The drawing under review shows one solid part. Ordinate dimensions are in mm from its lowest x, y, z. A direction names the side the tool comes from. Give positions to 0.01 mm unless a question says otherwise; leave off trailing zeros. Loops run counter-clockwise (first coordinate to the right, second up) from the corner with the lowest first, then second, coordinate; pieces in that order, holes last. Notation, with made-up numbers: (14, 46.5) -> (49, 46.5) arc R28 cw to (49, 76.5) -> close; hole circle Ø11 at (56, 83). An arc over 180 degrees is marked (long way). Answer in a Markdown table with one row per item. Add a question column.
(1) Draft analysis for pull direction X (two halves, no side actions). For the marked faces 3, 4 and 5, state which applies: +X half, -X half, draft (parallel to the pull), parting line (faces both ways), or undercut.
(2) Consider section B-B on x = 14.5. Write out the cut boundary in (y, z), then the cut area to 3 significant figures.
(3) Consider section A-A on z = 25. Write out the cut boundary in (x, y), then the cut area to 3 significant figures.
(4) For line 1 (Z direction, x = 9.5, y = 0.4); line 2 (Y direction, x = 7.5, z = 17); line 3 (X direction, y = 0.25, z = 25), list the stretches that pass through material, from the lowest coordinate up.
(5) For the marked faces 1 and 2, list the 3-axis set-ups (+Z, -Z, +X, -X, +Y, -Y) from which the entire face can be reached by the end or side of a thin tool; tool diameter is ignored.
(6) Consider section D-D on x = 9.5. Write out the cut boundary in (y, z).
(7) For pin 1 (8.5 mm diameter, centred on y = 6, z = 12.5, fed in from -X); pin 2 (5 mm diameter, centred on x = 5, y = 9, fed in from -Z), all flat-tipped, find the tip position at first contact; note any pin that passes through.
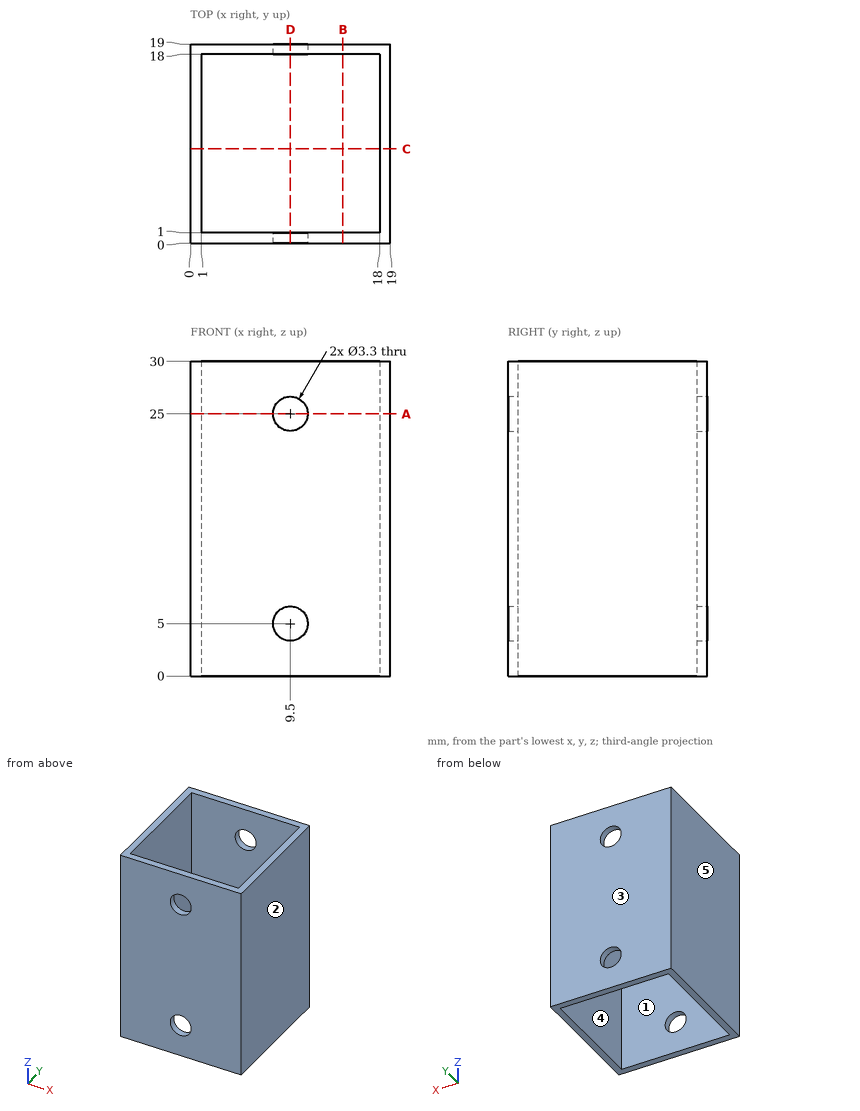
Values follow:
| question | item | result |
|---|---|---|
| 1 | face 3 | draft |
| 1 | face 4 | undercut |
| 1 | face 5 | -X half |
| 2 | outline | (0, 0) -> (1, 0) -> (1, 30) -> (0, 30) -> close; (18, 0) -> (19, 0) -> (19, 30) -> (18, 30) -> close |
| 2 | area | 60.0 mm2 |
| 3 | outline | (0, 0) -> (7.85, 0) -> (7.85, 1) -> (1, 1) -> (1, 18) -> (7.85, 18) -> (7.85, 19) -> (0, 19) -> close; (11.15, 0) -> (19, 0) -> (19, 19) -> (11.15, 19) -> (11.15, 18) -> (18, 18) -> (18, 1) -> (11.15, 1) -> close |
| 3 | area | 65.4 mm2 |
| 4 | line 1 | 0 to 3.35, 6.65 to 23.35, 26.65 to 30 |
| 4 | line 2 | 0 to 1, 18 to 19 |
| 4 | line 3 | 0 to 7.85, 11.15 to 19 |
| 5 | face 1 | +Z, -Z |
| 5 | face 2 | +Z, -Z, +X, +Y, -Y |
| 6 | outline | (0, 0) -> (1, 0) -> (1, 3.35) -> (0, 3.35) -> close; (0, 6.65) -> (1, 6.65) -> (1, 23.35) -> (0, 23.35) -> close; (0, 26.65) -> (1, 26.65) -> (1, 30) -> (0, 30) -> close; (18, 0) -> (19, 0) -> (19, 3.35) -> (18, 3.35) -> close; (18, 6.65) -> (19, 6.65) -> (19, 23.35) -> (18, 23.35) -> close; (18, 26.65) -> (19, 26.65) -> (19, 30) -> (18, 30) -> close |
| 7 | pin 1 | x = 0 |
| 7 | pin 2 | through |
